```python
from build123d import *

# Parameters (mm, degrees)
BOSS_EXTRUDE1_DEPTH = 1.8
BOSS_EXTRUDE3_DEPTH = 4
CUT_EXTRUDE1_DEPTH  = 51.248019596
FILLET1_R           = 4
FILLET2_R           = 0.3


with BuildPart() as part:
    # Sketch1 → Boss-Extrude1 (new body)
    with BuildSketch(Plane(origin=(0, 0, 0), x_dir=(1, 0, 0), z_dir=(0, 1, 0))):
        with BuildLine():
            ThreePointArc((-1.998520163, 25.923076923), (-18.384776311, 18.384776311), (-25.923076923, 1.998520163))
            ThreePointArc((-25.923076923, 1.998520163), (-28, 0), (-25.923076923, -1.998520163))
            ThreePointArc((-25.923076923, -1.998520163), (-18.384776311, -18.384776311), (-1.998520163, -25.923076923))
            ThreePointArc((-1.998520163, -25.923076923), (0, -28), (1.998520163, -25.923076923))
            ThreePointArc((1.998520163, -25.923076923), (18.384776311, -18.384776311), (25.923076923, -1.998520163))
            ThreePointArc((25.923076923, -1.998520163), (28, 0), (25.923076923, 1.998520163))
            ThreePointArc((25.923076923, 1.998520163), (18.384776311, 18.384776311), (1.998520163, 25.923076923))
            ThreePointArc((1.998520163, 25.923076923), (0, 28), (-1.998520163, 25.923076923))
        make_face()
        with BuildLine():
            Line((-18.466185313, 15.329709717), (18.466185313, 15.329709717))
            ThreePointArc((18.466185313, 15.329709717), (0, -24), (-18.466185313, 15.329709717))
        make_face(mode=Mode.SUBTRACT)
    extrude(amount=BOSS_EXTRUDE1_DEPTH)

    # Sketch2 → Boss-Extrude3 (add)
    with BuildSketch(Plane(origin=(0, 1.8, 0), x_dir=(1, 0, 0), z_dir=(0, 1, 0))):
        with BuildLine():
            Line((-13.318560882, 15.329709717), (13.318560882, 15.329709717))
            Line((13.318560882, 15.329709717), (13.318560882, 22.329709717))
            ThreePointArc((13.318560882, 22.329709717), (0, 26), (-13.318560882, 22.329709717))
            Line((-13.318560882, 22.329709717), (-13.318560882, 15.329709717))
        make_face()
    extrude(amount=BOSS_EXTRUDE3_DEPTH)

    # Sketch3 → Cut-Extrude1 (cut, through all)
    with BuildSketch(Plane.ZY.offset(13.318560882)):
        Polygon((-15.329709717, 5.8), (-19.329709717, 1.8), (-20.729709717, 1.8), (-16.729709717, 5.8), align=None)
    extrude(amount=-CUT_EXTRUDE1_DEPTH, mode=Mode.SUBTRACT)

    # Fillet1
    fillet1_edges = [part.edges().sort_by_distance(p)[0] for p in [
        (0, 5.8, -26),
    ]]
    fillet(fillet1_edges, radius=FILLET1_R - 0.0001)  # a hair under: the kernel refuses the full size

    # Fillet2
    fillet2_edges = [part.edges().sort_by_distance(p)[0] for p in [
        (0, 5.8, -15.329709717),
        (0, 5.8, -16.729709717),
    ]]
    fillet(fillet2_edges, radius=FILLET2_R)


solid = part.part
```
Check sheet for the modelled part. Datum: model origin and axes. Units: mm. A direction names the side the tool comes from. Round coordinates to 2 decimals unless told otherwise and drop trailing zeros. Order: outer loops, then holes, each group sorted by start corner. A loop starts at its lowest first (then second) coordinate and runs counter-clockwise, first axis right, second up. Notation, with made-up numbers: (73.25, 45.5) - (81.25, 45.5) arc R13 ccw to (81.25, 55.5) - close; hole circle Ø6 at (-0.5, 56.5). An arc over 180 degrees is marked (long way). Write item = value, one per line.
Q1. Section check D-D (y = 3.45). Record the boundary of the cut face in (x, z), and give its area (3 significant figures).
Computed:
outline = (-13.32, -21.91) arc R25.64 ccw to (13.32, -21.91) - (13.32, -19.08) - (-13.32, -19.08) - close; (-13.32, -17.68) - (13.32, -17.68) - (13.32, -15.33) - (-13.32, -15.33) - close
area = 205 mm^2
Q2. Section check C-C (y = 0.65). Record the boundary of the cut face in (x, z).
Computed:
outline = (-25.92, -2) arc R26 ccw to (-2, -25.92) arc R2 ccw (long way) to (2, -25.92) arc R26 ccw to (25.92, -2) arc R2 ccw (long way) to (25.92, 2) arc R26 ccw to (2, 25.92) arc R2 ccw (long way) to (-2, 25.92) arc R26 ccw to (-25.92, 2) arc R2 ccw (long way) to start; hole (-18.47, -15.33) - (18.47, -15.33) arc R24 ccw (long way) to start
Q3. Section check A-A (z = 0). Record the boundary of the cut face in (x, y), and give its area (3 significant figures).
Computed:
outline = (-28, 0) - (-24, 0) - (-24, 1.8) - (-28, 1.8) - close; (24, 0) - (28, 0) - (28, 1.8) - (24, 1.8) - close
area = 14.4 mm^2
Q4. Tool access check on faces 1 (the face through (-13.319, 3, -17)), 2 (the face through (13.319, 3, -17)), 3 (the face through (-0.19, 3.52, -19.01)). Record the directions out of +Z, -Z, +X, -X, +Y, -Y that give a thin tool (end or side, any length) a straight path to the whole face; none if there is none.
Computed:
face_1 = +Z, -Z, -X, +Y
face_2 = +Z, -Z, +X, +Y
face_3 = +X, -X
Q5. Thickness scan on line 1 along X through (y, z) = (0.95, 18); line 2 along Z through (x, y) = (7, 1.55); line 3 along Y through (x, z) = (13, -20.5). Record the ranges inside material, lowest first.
Computed:
line_1 = -18.76 to -15.87, 15.87 to 18.76
line_2 = -25.04 to -15.33, 22.96 to 25.04
line_3 = 0 to 1.8, 2.03 to 5.09
Q6. Draft check along X on faces 4 (the face through (18.2, 0.89, 18.57)), 5 (the face through (-0.19, 3.57, -17.56)), 6 (the face through (0, 3, -15.33)). Enter one of: pulls with the +X half, pulls with the -X half, needs draft (parallel to the pull), parting line crosses it, or undercut.
Computed:
face_4 = pulls with the +X half
face_5 = needs draft
face_6 = undercut
Q7. Go/stop test with flat-tipped pins: pin 1 (1.5 mm diameter, centred on x = -18.5, y = 4, fed in from +Z); pin 2 (1.5 mm diameter, centred on x = -8.5, y = 3.5, fed in from +Z); pin 3 (0.6 mm diameter, centred on x = -1, z = -27.5, fed in from +Y); pin 4 (3 mm diameter, centred on y = 3, z = -16.5, fed in from +X). Record where each tip stops, or that it passes through.
Computed:
pin_1 = through
pin_2 = -15.33
pin_3 = 1.8
pin_4 = 20.8
